Here's how the part is built. I have some questions about the finished solid (model axes, mm). Face numbers are marked on the shaded views. A direction names the side the tool comes from. Round coordinates to 2 decimals unless told otherwise and drop trailing zeros. Loops run counter-clockwise (first coordinate to the right, second up) from the corner with the lowest first, then second, coordinate; pieces in that order, holes last. Notation, with made-up numbers: (-3.5, 14) -> (26.5, 14) arc R33 cw to (26.5, 43) -> close; hole circle Ø10 at (-19.75, 85.25). An arc over 180 degrees is marked (long way). One line per item, written item: value. Start each with the question number.
```python
from build123d import *

# Parameters (mm, degrees)
SKETCH1_W           = 7
SKETCH1_H           = 1.46
BOSS_EXTRUDE1_DEPTH = 2
SKETCH2_W           = 8
SKETCH2_H           = 8
BOSS_EXTRUDE2_DEPTH = 11.74993
BOSS_EXTRUDE3_DEPTH = 1.6
SKETCH4_R           = 7.7
BOSS_EXTRUDE4_DEPTH = 7.5
SKETCH5_R           = 6.95
CUT_EXTRUDE1_DEPTH  = 7.5
CUT_EXTRUDE2_DEPTH  = 7.5
CIRPATTERN1_COUNT   = 4


with BuildPart() as part:
    # Sketch1 → Boss-Extrude1 (new body)
    with BuildSketch(Plane.XY):
        with BuildLine():
            Line((-11.7, 4), (11.7, 4))
            ThreePointArc((11.7, 4), (13.821320344, 3.121320344), (14.7, 1))
            Line((14.7, 1), (14.7, -1))
            ThreePointArc((14.7, -1), (13.821320344, -3.121320344), (11.7, -4))
            Line((11.7, -4), (-11.7, -4))
            ThreePointArc((-11.7, -4), (-13.821320344, -3.121320344), (-14.7, -1))
            Line((-14.7, -1), (-14.7, 1))
            ThreePointArc((-14.7, 1), (-13.821320344, 3.121320344), (-11.7, 4))
        make_face()
        with Locations((-8.5, 0)):
            Rectangle(SKETCH1_W, SKETCH1_H, mode=Mode.SUBTRACT)
        with Locations((8.5, 0)):
            Rectangle(SKETCH1_W, SKETCH1_H, mode=Mode.SUBTRACT)
    extrude(amount=BOSS_EXTRUDE1_DEPTH)

    # Sketch2 → Boss-Extrude2 (add)
    with BuildSketch(Plane.XY):
        Rectangle(SKETCH2_W, SKETCH2_H)
    extrude(amount=BOSS_EXTRUDE2_DEPTH)

    # Sketch3 → Boss-Extrude3 (add)
    with BuildSketch(Plane.XY.offset(11.74993)):
        with BuildLine():
            Line((-5.05, 9.000108401), (5.05, 9.000108401))
            ThreePointArc((5.05, 9.000108401), (7.878427125, 7.828535526), (9.05, 5.000108401))
            Line((9.05, 5.000108401), (9.05, -5.000108401))
            ThreePointArc((9.05, -5.000108401), (7.878427125, -7.828535526), (5.05, -9.000108401))
            Line((5.05, -9.000108401), (-5.05, -9.000108401))
            ThreePointArc((-5.05, -9.000108401), (-7.878427125, -7.828535526), (-9.05, -5.000108401))
            Line((-9.05, -5.000108401), (-9.05, 5.000108401))
            ThreePointArc((-9.05, 5.000108401), (-7.878427125, 7.828535526), (-5.05, 9.000108401))
        make_face()
    extrude(amount=BOSS_EXTRUDE3_DEPTH)

    # Sketch4 → Boss-Extrude4 (add)
    with BuildSketch(Plane.XY.offset(13.34993)):
        Circle(SKETCH4_R)
    extrude(amount=BOSS_EXTRUDE4_DEPTH)

    # Sketch5 → Cut-Extrude1 (cut)
    with BuildSketch(Plane.XY.offset(13.34993)):
        Circle(SKETCH5_R)
    extrude(amount=CUT_EXTRUDE1_DEPTH, mode=Mode.SUBTRACT)

    # Sketch11 → Cut-Extrude2 (cut)
    with BuildSketch(Plane.XY.offset(13.34993)):
        Polygon((0, 8.183776361), (-0.55, 8.183776361), (0, 0), (0.55, 8.183776361), align=None)
    cut_extrude2 = extrude(amount=CUT_EXTRUDE2_DEPTH, mode=Mode.SUBTRACT)

    # CirPattern1: Cut-Extrude2 ×4 about axis
    cirpattern1_axis = Axis((0, 0, 20.84993), (0, 0, -1))
    for i in range(1, CIRPATTERN1_COUNT):
        add(cut_extrude2.rotate(cirpattern1_axis, i * 360 / CIRPATTERN1_COUNT), mode=Mode.SUBTRACT)


solid = part.part
```
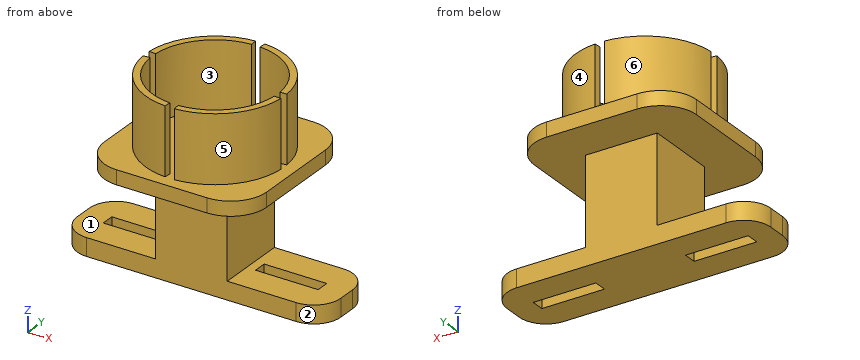
Q1. I want a section at D-D on y = -1.75. Please give me the cut outline in (x, z), plus the area to 3 significant figures.
Q2. If we mould it in two halves opening along Y, with no side actions, what happens to the marked faces 1, 2 and 3? For each: released by +Y, released by -Y, zero draft, split by the parting line, or undercut.
Q3. Which directions (+Z, -Z, +X, -X, +Y, -Y) give clear straight access to the entire face, cutting with the end or side of a thin tool? Please do the marked faces 4, 5 and 6.
Q4. If I drill on line 1 along Z through (x, y) = (6.25, 1.75); line 2 along X through (y, z) = (3, 9.5); line 3 along Z through (x, y) = (-10.5, 3.5), over which ranges is the centre line in solid material (lowest first)?
Q5. I want a section at C-C on x = 6.5. Please give me the cut outline in (y, z).
Q6. Will these pins go through, and if not, where does the flat tip stop? P1, Ø3, axis at x = -1.5, z = 9.5, coming from the -Y side; P2, Ø2.5, axis at y = -1, z = 9, coming from the -X side; P3, Ø4, axis at y = 0.5, z = 5, coming from the +X side.
Q7. I want a section at A-A on x = 10.25. Please give me the cut outline in (y, z).
Q8. I want a section at B-B on z = 19.5. Please give me the cut outline in (x, y), plus the area to 3 significant figures.
Answers below:
1. outline: (-14.6, 0) -> (14.6, 0) -> (14.6, 2) -> (4, 2) -> (4, 11.75) -> (9.05, 11.75) -> (9.05, 13.35) -> (7.5, 13.35) -> (7.5, 20.85) -> (6.73, 20.85) -> (6.73, 13.35) -> (-6.73, 13.35) -> (-6.73, 20.85) -> (-7.5, 20.85) -> (-7.5, 13.35) -> (-9.05, 13.35) -> (-9.05, 11.75) -> (-4, 11.75) -> (-4, 2) -> (-14.6, 2) -> close
1. area: 177 mm^2
2. face 1: zero draft
2. face 2: released by -Y
2. face 3: undercut
3. face 4: +Z, +X, +Y
3. face 5: +Z, +X, -Y
3. face 6: +Z, -X, +Y
4. line 1: z = 0 to 2, 11.75 to 13.35
4. line 2: x = -4 to 4
4. line 3: z = 0 to 2
5. outline: (-8.73, 11.75) -> (8.73, 11.75) -> (8.73, 13.35) -> (4.13, 13.35) -> (4.13, 20.85) -> (2.46, 20.85) -> (2.46, 13.35) -> (-2.46, 13.35) -> (-2.46, 20.85) -> (-4.13, 20.85) -> (-4.13, 13.35) -> (-8.73, 13.35) -> close; (-4, 0) -> (-0.73, 0) -> (-0.73, 2) -> (-4, 2) -> close; (0.73, 0) -> (4, 0) -> (4, 2) -> (0.73, 2) -> close
6. P1: stops at y = -4
6. P2: stops at x = -4
6. P3: stops at x = 4
7. outline: (-4, 0) -> (-0.73, 0) -> (-0.73, 2) -> (-4, 2) -> close; (0.73, 0) -> (4, 0) -> (4, 2) -> (0.73, 2) -> close
8. outline: (-7.68, -0.52) arc R7.7 ccw to (-0.52, -7.68) -> (-0.47, -6.93) arc R6.95 cw to (-6.93, -0.47) -> close; (-7.68, 0.52) -> (-6.93, 0.47) arc R6.95 cw to (-0.47, 6.93) -> (-0.52, 7.68) arc R7.7 ccw to start; (0.47, -6.93) -> (0.52, -7.68) arc R7.7 ccw to (7.68, -0.52) -> (6.93, -0.47) arc R6.95 cw to start; (0.47, 6.93) arc R6.95 cw to (6.93, 0.47) -> (7.68, 0.52) arc R7.7 ccw to (0.52, 7.68) -> close
8. area: 31.6 mm^2
